```python
from build123d import *

# Parameters (mm, degrees)
F1_DEPTH   = 21.6836184263
F2_R       = 20.8194643485
F3_DEPTH   = 14.0719488263
F7_D       = 6.35
F7_DEPTH   = 14.0729488263
F7_ON_F6_D = 6.35


# Not quite as in the source:
# - the program builds the solid bodies; features that only make, move or delete a surface that nothing else refers to are left out


with BuildPart() as f1:
    # F0 (on Top) → F1 (new body)
    with BuildSketch(Plane.XY):
        Polygon((50.926592201, 50.2595603466), (-46.1172051728, 50.2595603466), (-46.1172051728, -50.9577989578), (50.926592201, -50.9577989578), (50.926592201, 48.6862957478), align=None)
    extrude(amount=F1_DEPTH)

    # F2 (on face) → F3 (join)
    with BuildSketch(Plane.XY.offset(21.6836184263)):
        with Locations((0, -6.2367771752)):
            Circle(F2_R)
    extrude(amount=F3_DEPTH)

    # F7 (through all, one way)
    with BuildSketch(Plane(origin=(0, 0, 21.6836184263), x_dir=(1, 0, 0), z_dir=(0, 0, -1))):
        with Locations((0, 6.2367771752)):
            Circle(F7_D / 2)
    extrude(amount=-F7_DEPTH, mode=Mode.SUBTRACT)

    # F7 on F6 (through all)
    with Locations(Plane(origin=(0, 0, 0), x_dir=(1, 0, 0), z_dir=(0, 0, -1))):
        with Locations((-8.5173435509, 0)):
            Hole(F7_ON_F6_D / 2)


solid = f1.part
```
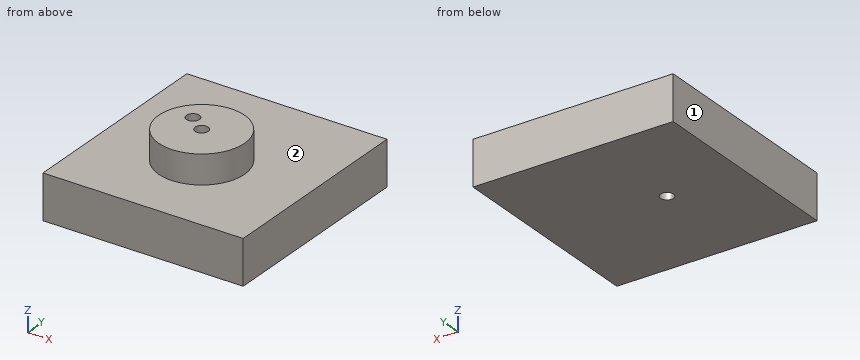
The model under review builds one solid part; all positions refer to its coordinate system, in mm. Face numbers are marked on the shaded views. A direction names the side the tool comes from. Round coordinates to 2 decimals unless told otherwise and drop trailing zeros. Loops run counter-clockwise (first coordinate to the right, second up) from the corner with the lowest first, then second, coordinate; pieces in that order, holes last.
1) Clearance check with flat-ended pins moving along their axes: P1, Ø5.5, axis at x = 0, y = -6.24, coming from the +Z side; P2, Ø10, axis at x = -11.5, z = 30.5, coming from the +Y side; P3, Ø1, axis at x = -7, z = 26.5, coming from the -Y side. State where each tip first meets the part, or that it passes through.
Values follow:
P1: stops at z = 21.68
P2: stops at y = 13.54
P3: stops at y = -26.02
2) Consider section A-A on y = 0. State the section outline as (x, z) points.
Values follow:
outline: (-46.12, 0) - (-11.69, 0) - (-11.69, 35.76) - (-19.86, 35.76) - (-19.86, 21.68) - (-46.12, 21.68) - close; (-5.34, 0) - (50.93, 0) - (50.93, 21.68) - (19.86, 21.68) - (19.86, 35.76) - (-5.34, 35.76) - close
3) Tool access review of the marked faces 1 and 2: name each direction out of +Z, -Z, +X, -X, +Y, -Y from which nothing blocks a thin tool from reaching the whole face with its end or side.
Values follow:
face 1: +Z, -Z, -X, +Y, -Y
face 2: +Z
4) Consider section B-B on x = 0. State the section outline as (y, z) points, then the cut area to 3 significant figures.
Values follow:
outline: (-50.96, 0) - (50.26, 0) - (50.26, 21.68) - (14.58, 21.68) - (14.58, 35.76) - (-3.06, 35.76) - (-3.06, 21.68) - (-9.41, 21.68) - (-9.41, 35.76) - (-27.06, 35.76) - (-27.06, 21.68) - (-50.96, 21.68) - close
area: 2,690 mm2
5) Wall thickness on line 1 along Y through (x, z) = (0, 30); line 2 along Z through (x, y) = (-7, 37.5); line 3 along Y through (x, z) = (-6, 2): over which ranges is each line inside the solid? List them lowest first.
Values follow:
line 1: y = -27.06 to -9.41, -3.06 to 14.58
line 2: z = 0 to 21.68
line 3: y = -50.96 to -1.93, 1.93 to 50.26
6) Consider section C-C on y = -18. State the section outline as (x, z) points, then the cut area to 3 significant figures.
Values follow:
outline: (-46.12, 0) - (50.93, 0) - (50.93, 21.68) - (17.18, 21.68) - (17.18, 35.76) - (-17.18, 35.76) - (-17.18, 21.68) - (-46.12, 21.68) - close
area: 2,590 mm2
7) Consider section D-D on z = 24. State the section outline as (x, y) points (3 decimals), then the cut area to 3 significant figures.
Values follow:
outline: circle Ø41.639 at (0, -6.237); hole circle Ø6.35 at (-8.517, 0); hole circle Ø6.35 at (0, -6.237)
area: 1,300 mm2
